The model under review builds one solid part; all positions refer to its coordinate system, in mm. A direction names the side the tool comes from. Coordinates: 2 decimals unless noted, no trailing zeros. Loops run counter-clockwise (first coordinate to the right, second up) from the corner with the lowest first, then second, coordinate; pieces in that order, holes last. Notation, with made-up numbers: (51.25, 88) - (95.25, 88) arc R13 ccw to (95.25, 92) - close; hole circle Ø10 at (-5, 55). An arc over 180 degrees is marked (long way). Use a Markdown table: item, result. Add a question column.
1) Clearance check with flat-ended pins moving along their axes: pin 1 (6 mm diameter, centred on x = 8.5, z = 95, fed in from +Y); pin 2 (10 mm diameter, centred on x = 15, z = 34, fed in from -Y); pin 3 (6 mm diameter, centred on x = 14, y = -96, fed in from +Z). State where each tip first meets the part, or that it passes through.
2) For faces 1 (the flat face through (10, -84.905, 31)), 2 (the flat face through (10, -95, 40.937)), 3 (the flat face through (10, -95, 120.937)), 4 (the flat face through (10, -224.905, 71)), 5 (the flat face through (10, -235, 40.937)), list the 3-axis set-ups (+Z, -Z, +X, -X, +Y, -Y) from which the entire face can be reached by the end or side of a thin tool; tool diameter is ignored.
3) The part is to be moulded in two halves that separate along Z. For faces 6 (the flat face through (10, -95, 60.937)), 7 (the flat face through (10, -244.905, 51)), 8 (the flat face through (10, -176, 140.937)), say which applies: pulls with the +Z half, pulls with the -Z half, needs draft (parallel to the pull), parting line crosses it, or undercut.
4) Add section A-A, the plane y = -228.5. Give the boundary of the cut face in (x, z), and give its area (3 significant figures).
5) To check wall thickness, follow L1, parallel to Z at x = 15, y = -229.5; L2, parallel to Y at x = 7.5, z = 83; L3, parallel to Y at x = 11.5, z = 62. State the ranges of each line that lie inside material, in increasing order. Write a range as [from, to].
6) Add section C-C, the plane z = 132. Give the boundary of the cut face in (x, y), and give its area (3 significant figures).
7) Add section B-B, the plane x = 12.25. Give the boundary of the cut face in (y, z).
```python
from build123d import *

# Parameters (mm, degrees)
F0_W      = 160
F0_H      = 120
F1_DEPTH  = 20
F2_W      = 20
F2_H      = 20
F3_DEPTH  = 20
F4_W      = 20
F4_H      = 20
F5_DEPTH  = 20
F6_W      = 20
F6_H      = 20
F7_DEPTH  = 20
F8_W      = 20
F8_H      = 20
F9_DEPTH  = 20
F10_W     = 20
F10_H     = 20
F11_DEPTH = 20
F12_W     = 20
F12_H     = 20
F13_DEPTH = 20


with BuildPart() as f1:
    # F0 (on Right) → F1 (new body)
    with BuildSketch(Plane.YZ):
        with Locations((-164.905177, 80.936906)):
            Rectangle(F0_W, F0_H)
    extrude(amount=F1_DEPTH)

    # F2 (on face) → F3 (cut)
    with BuildSketch(Plane.YZ.offset(20)):
        with Locations((-234.905177, 110.936906)):
            Rectangle(F2_W, F2_H)
    extrude(amount=-F3_DEPTH, mode=Mode.SUBTRACT)

    # F4 (on face) → F5 (cut)
    with BuildSketch(Plane.YZ.offset(20)):
        with Locations((-234.905177, 70.936906)):
            Rectangle(F4_W, F4_H)
    extrude(amount=-F5_DEPTH, mode=Mode.SUBTRACT)

    # F6 (on face) → F7 (cut)
    with BuildSketch(Plane.YZ.offset(20)):
        with Locations((-234.905177, 30.936906)):
            Rectangle(F6_W, F6_H)
    extrude(amount=-F7_DEPTH, mode=Mode.SUBTRACT)

    # F8 (on face) → F9 (cut)
    with BuildSketch(Plane.YZ.offset(20)):
        with Locations((-94.905177, 130.936906)):
            Rectangle(F8_W, F8_H)
    extrude(amount=-F9_DEPTH, mode=Mode.SUBTRACT)

    # F10 (on face) → F11 (cut)
    with BuildSketch(Plane.YZ.offset(20)):
        with Locations((-94.905177, 90.936906)):
            Rectangle(F10_W, F10_H)
    extrude(amount=-F11_DEPTH, mode=Mode.SUBTRACT)

    # F12 (on face) → F13 (cut)
    with BuildSketch(Plane.YZ.offset(20)):
        with Locations((-94.905177, 50.936906)):
            Rectangle(F12_W, F12_H)
    extrude(amount=-F13_DEPTH, mode=Mode.SUBTRACT)


solid = f1.part
```
From the geometry:
| question | item | result |
|---|---|---|
| 1 | pin 1 | stops at y = -104.91 |
| 1 | pin 2 | stops at y = -224.91 |
| 1 | pin 3 | stops at z = 120.94 |
| 2 | face 1 | +Z, -Z, +X, -X, +Y |
| 2 | face 2 | +X, -X, +Y |
| 2 | face 3 | +Z, +X, -X, +Y |
| 2 | face 4 | +X, -X, -Y |
| 2 | face 5 | -Z, +X, -X, -Y |
| 3 | face 6 | undercut |
| 3 | face 7 | needs draft |
| 3 | face 8 | pulls with the +Z half |
| 4 | outline | (0, 40.94) - (20, 40.94) - (20, 60.94) - (0, 60.94) - close; (0, 80.94) - (20, 80.94) - (20, 100.94) - (0, 100.94) - close; (0, 120.94) - (20, 120.94) - (20, 140.94) - (0, 140.94) - close |
| 4 | area | 1,200 mm^2 |
| 5 | L1 | z = [40.94, 60.94], [80.94, 100.94], [120.94, 140.94] |
| 5 | L2 | y = [-244.91, -104.91] |
| 5 | L3 | y = [-224.91, -84.91] |
| 6 | outline | (0, -244.91) - (20, -244.91) - (20, -104.91) - (0, -104.91) - close |
| 6 | area | 2,800 mm^2 |
| 7 | outline | (-244.91, 40.94) - (-224.91, 40.94) - (-224.91, 20.94) - (-84.91, 20.94) - (-84.91, 40.94) - (-104.91, 40.94) - (-104.91, 60.94) - (-84.91, 60.94) - (-84.91, 80.94) - (-104.91, 80.94) - (-104.91, 100.94) - (-84.91, 100.94) - (-84.91, 120.94) - (-104.91, 120.94) - (-104.91, 140.94) - (-244.91, 140.94) - (-244.91, 120.94) - (-224.91, 120.94) - (-224.91, 100.94) - (-244.91, 100.94) - (-244.91, 80.94) - (-224.91, 80.94) - (-224.91, 60.94) - (-244.91, 60.94) - close |
